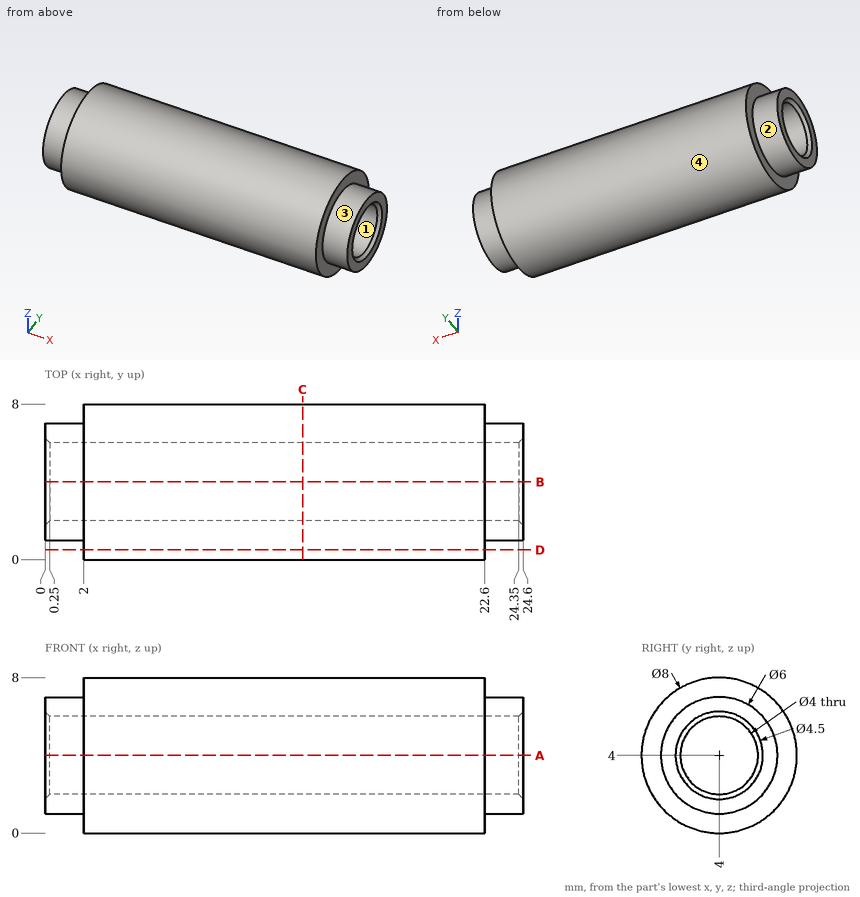
For this review, use the dimensioned drawing (mm, ordinates from the lowest corner) and the shaded views. A direction names the side the tool comes from. Coordinates: 2 decimals unless noted, no trailing zeros. Loops run counter-clockwise (first coordinate to the right, second up) from the corner with the lowest first, then second, coordinate; pieces in that order, holes last. Notation, with made-up numbers: (87.25, 30.25) -> (115.25, 30.25) arc R9 ccw to (115.25, 39.25) -> close; hole circle Ø3 at (-2.5, 18). An arc over 180 degrees is marked (long way). Use a Markdown table: item, result. Add a question column.
Item 1: We need section A-A, the plane z = 4. Write out the cut boundary in (x, y).
Item 2: Machinability: for the marked faces 3 and 4, which of the approach directions +Z, -Z, +X, -X, +Y, -Y give a long, thin tool a straight path to every point of the face, cutting with its end or side? Answer none if there is none.
Item 3: We need section D-D, the plane y = 0.5. Write out the cut boundary in (x, z), and give its area (3 significant figures).
Item 4: We need section C-C, the plane x = 13.25. Write out the cut boundary in (y, z), and give its area (3 significant figures).
Item 5: Wall thickness on L1, parallel to Y at x = 18.75, z = 4; L2, parallel to X at y = 7.25, z = 4; L3, parallel to Y at x = 5, z = 3.25: over which ranges is each line inside the solid? List them lowest first. Write a range as from..to.
Item 6: Clearance check with flat-ended pins moving along their axes: P1, Ø3, axis at x = 20.5, z = 6, coming from the -Y side; P2, Ø1, axis at x = 14, y = 2.5, coming from the -Z side; P3, Ø1, axis at x = 5, y = 1.5, coming from the +Z side. State where each tip first meets the part, or that it passes through.
Item 7: The part is to be moulded in two halves that separate along Z. For the marked faces 1 and 2, say which applies: +Z half, -Z half, draft (parallel to the pull), parting line (faces both ways), or undercut.
Numbers:
| question | item | result |
|---|---|---|
| 1 | outline | (0, 1) -> (2, 1) -> (2, 0) -> (22.6, 0) -> (22.6, 1) -> (24.6, 1) -> (24.6, 1.75) -> (24.35, 2) -> (0.25, 2) -> (0, 1.75) -> close; (0, 6.25) -> (0.25, 6) -> (24.35, 6) -> (24.6, 6.25) -> (24.6, 7) -> (22.6, 7) -> (22.6, 8) -> (2, 8) -> (2, 7) -> (0, 7) -> close |
| 2 | face 3 | +X |
| 2 | face 4 | +X, -X |
| 3 | outline | (2, 2.06) -> (22.6, 2.06) -> (22.6, 5.94) -> (2, 5.94) -> close |
| 3 | area | 79.8 mm^2 |
| 4 | outline | circle Ø8 at (4, 4); hole circle Ø4 at (4, 4) |
| 4 | area | 37.7 mm^2 |
| 5 | L1 | y = 0..2, 6..8 |
| 5 | L2 | x = 2..22.6 |
| 5 | L3 | y = 0.07..2.15, 5.85..7.93 |
| 6 | P1 | stops at y = 0.03 |
| 6 | P2 | stops at z = 0.13 |
| 6 | P3 | stops at z = 7.46 |
| 7 | face 1 | undercut |
| 7 | face 2 | parting line |
